```python
from build123d import *

# Parameters (mm, degrees)
SKETCH1_W           = 20.32
SKETCH1_H           = 20.32
BOSS_EXTRUDE1_DEPTH = 20.32
SKETCH2_R           = 4.675
CUT_EXTRUDE1_DEPTH  = 10.1
CIRPATTERN1_COUNT   = 4


with BuildPart() as part:
    # Sketch1 → Boss-Extrude1 (new body)
    with BuildSketch(Plane(origin=(0, 0, 0), x_dir=(1, 0, 0), z_dir=(0, 1, 0))):
        Rectangle(SKETCH1_W, SKETCH1_H)
    extrude(amount=BOSS_EXTRUDE1_DEPTH)

    # Sketch2 → Cut-Extrude1 (cut)
    with BuildSketch(Plane.XY.offset(10.16)):
        with Locations((0, 10.16)):
            Circle(SKETCH2_R)
    cut_extrude1 = extrude(amount=-CUT_EXTRUDE1_DEPTH, mode=Mode.SUBTRACT)

    # CirPattern1: Cut-Extrude1 ×4 about axis
    cirpattern1_axis = Axis((0, 0, 0), (0, 1, 0))
    for i in range(1, CIRPATTERN1_COUNT):
        add(cut_extrude1.rotate(cirpattern1_axis, i * 360 / CIRPATTERN1_COUNT), mode=Mode.SUBTRACT)


solid = part.part
```
Geometry: final body of the model. Coordinates: model frame, mm. Coordinates: 2 decimals unless noted, no trailing zeros. Order: outer loops, then holes, each group sorted by start corner. A loop starts at its lowest first (then second) coordinate and runs counter-clockwise, first axis right, second up. Notation, with made-up numbers: M 51,38 L 106,38 A19 cw 106,54 Z; hole C 55.5,29.25 d7. An arc over 180 degrees is marked long. Answer in a Markdown table with one row per item. Add a question column.
Q1. Mould query, pull axis Y, two halves, no side actions, for faces 1 (the cylindrical face through (3.446, 13.32, -6.303)), 2 (the cylindrical face through (-3.446, 13.32, 6.303)), 3 (the flat face through (0, 0, 0)), 4 (the flat face through (-5, 8, 10.16)). Classes: released by +Y, released by -Y, zero draft, split by the parting line, or undercut.
Q2. Section query B-B on y = 10.16. Return the cut outline in (x, z) (3 decimals), and give its area (3 significant figures).
Q3. Line query: L1, parallel to Y at x = -6.5, z = 0 (3 decimals); L2, parallel to Z at x = -5, y = 10.16 (3 decimals). Output: solid intervals per line, ascending.
Q4. Section query A-A on x = -6. Return the cut outline in (y, z) (3 decimals), and give its area (3 significant figures).
Q5. Section query D-D on x = 1.75. Return the cut outline in (y, z) (3 decimals), and give its area (3 significant figures).
Q6. Contact query for a flat-ended pin moving along its axis: P1, Ø2, axis at x = -3, y = 11.5, coming from the -Z side. Output: stop coordinate, or through.
Q7. Section query C-C on z = -6.25. Return the cut outline in (x, y) (3 decimals), and give its area (3 significant figures).
Completed:
| question | item | result |
|---|---|---|
| 1 | face 1 | undercut |
| 1 | face 2 | undercut |
| 1 | face 3 | released by -Y |
| 1 | face 4 | zero draft |
| 2 | outline | M -10.16,-10.16 L -4.675,-10.16 L -4.675,-4.675 L -10.16,-4.675 Z; M -10.16,4.675 L -4.675,4.675 L -4.675,10.16 L -10.16,10.16 Z; M -0.06,-0.06 L 0.06,-0.06 L 0.06,0.06 L -0.06,0.06 Z; M 4.675,-10.16 L 10.16,-10.16 L 10.16,-4.675 L 4.675,-4.675 Z; M 4.675,4.675 L 10.16,4.675 L 10.16,10.16 L 4.675,10.16 Z |
| 2 | area | 120 mm2 |
| 3 | L1 | y = 0 to 5.485, 14.835 to 20.32 |
| 3 | L2 | z = -10.16 to -4.675, 4.675 to 10.16 |
| 4 | outline | M 0,-10.16 L 20.32,-10.16 L 20.32,10.16 L 0,10.16 Z; hole C 10.16,0 d9.35 |
| 4 | area | 344 mm2 |
| 5 | outline | M 0,-10.16 L 5.825,-10.16 L 5.825,-1.75 A4.675 cw 5.825,1.75 L 5.825,10.16 L 0,10.16 Z; M 14.495,-10.16 L 20.32,-10.16 L 20.32,10.16 L 14.495,10.16 L 14.495,1.75 A4.675 cw 14.495,-1.75 Z |
| 5 | area | 235 mm2 |
| 6 | P1 | passes through |
| 7 | outline | M -10.16,0 L 10.16,0 L 10.16,20.32 L -10.16,20.32 Z; hole C 0,10.16 d9.35 |
| 7 | area | 344 mm2 |
